```python
from build123d import *

# Parameters (mm, degrees)
SKETCH1_W           = 22.225
SKETCH1_H           = 17.4625
BOSS_EXTRUDE1_DEPTH = 50.8
CUT_EXTRUDE1_REACH  = 60.134
SKETCH2_R           = 2.032


with BuildPart() as part:
    # Sketch1 → Boss-Extrude1 (new body)
    with BuildSketch(Plane.XY):
        with Locations((11.1125, 8.73125)):
            Rectangle(SKETCH1_W, SKETCH1_H)
    extrude(amount=BOSS_EXTRUDE1_DEPTH)

    # Sketch2 → Cut-Extrude1 (cut, up to next)
    with BuildSketch(Plane.XZ, mode=Mode.PRIVATE) as cut_extrude1_sk1:
        with Locations(Location((11.1125, 44.45, 0), (0, 0, 270))):
            Circle(SKETCH2_R)
    cut_extrude1_tool1 = extrude(cut_extrude1_sk1.sketch, amount=-CUT_EXTRUDE1_REACH, mode=Mode.PRIVATE) & part.part
    # Sketch2 → Cut-Extrude1 (cut, up to next)
    with BuildSketch(Plane.XZ, mode=Mode.PRIVATE) as cut_extrude1_sk2:
        with Locations(Location((11.1125, 6.35, 0), (0, 0, 270))):
            Circle(SKETCH2_R)
    cut_extrude1_tool2 = extrude(cut_extrude1_sk2.sketch, amount=-CUT_EXTRUDE1_REACH, mode=Mode.PRIVATE) & part.part
    # Sketch2 → Cut-Extrude1 (cut, up to next)
    with BuildSketch(Plane.XZ, mode=Mode.PRIVATE) as cut_extrude1_sk3:
        Polygon((14.998644662, 25.4), (13.055572331, 28.7655), (9.169427669, 28.7655), (7.226355338, 25.4), (9.169427669, 22.0345), (13.055572331, 22.0345), align=None)
    cut_extrude1_tool3 = extrude(cut_extrude1_sk3.sketch, amount=-CUT_EXTRUDE1_REACH, mode=Mode.PRIVATE) & part.part
    add(cut_extrude1_tool1.solids().sort_by_distance((11.1125, 0, 44.45))[0], mode=Mode.SUBTRACT)
    add(cut_extrude1_tool2.solids().sort_by_distance((11.1125, 0, 6.35))[0], mode=Mode.SUBTRACT)
    add(cut_extrude1_tool3.solids().sort_by_distance((11.1125, 0, 25.4))[0], mode=Mode.SUBTRACT)


solid = part.part
```
Geometry check sheet. Reference: the model listing, model coordinates, mm. A direction names the side the tool comes from. Round coordinates to 2 decimals unless told otherwise and drop trailing zeros. Order: outer loops, then holes, each group sorted by start corner. A loop starts at its lowest first (then second) coordinate and runs counter-clockwise, first axis right, second up. Notation, with made-up numbers: (57.25, -20) - (74.25, -20) arc R26 cw to (74.25, -1) - close; hole circle Ø10 at (56, -4.5). An arc over 180 degrees is marked (long way). Use a Markdown table: item, result. Add a question column.
(1) Sectioned sample at B-B, the plane z = 6.35. Enter the section's corners in (x, y) (1 decimal), and give its area (3 significant figures).
(2) Material ranges on line 1 along Z through (x, y) = (11.25, 16); line 2 along X through (y, z) = (6.25, 6.35) (1 decimal); line 3 along Z through (x, y) = (9.5, 12.5), recorded low to high. Write a range as [from, to].
(3) Release check for a two-part mould opening along Z. For faces 1 (the flat face through (11, 9, 0)), 2 (the flat face through (0, 9, 25)), 3 (the flat face through (14.04, 8.61, 27.06)) record: pulls with the +Z half, pulls with the -Z half, needs draft (parallel to the pull), parting line crosses it, or undercut.
(4) Tool access check on faces 4 (the flat face through (22.225, 9, 25)), 5 (the flat face through (11, 9, 28.766)). Record the directions out of +Z, -Z, +X, -X, +Y, -Y that give a thin tool (end or side, any length) a straight path to the whole face; none if there is none.
(5) Sectioned sample at C-C, the plane y = 2.75. Count the separate pieces of the cut face and the enclosed holes in it, and give its area (3 significant figures).
(6) Sectioned sample at A-A, the plane x = 8. Enter the section's corners in (y, z).
Answers below:
| question | item | result |
|---|---|---|
| 1 | outline | (0, 0) - (9.1, 0) - (9.1, 17.5) - (0, 17.5) - close; (13.1, 0) - (22.2, 0) - (22.2, 17.5) - (13.1, 17.5) - close |
| 1 | area | 317 mm² |
| 2 | line 1 | [0, 4.32], [8.38, 22.03], [28.77, 42.42], [46.48, 50.8] |
| 2 | line 2 | [0, 9.1], [13.1, 22.2] |
| 2 | line 3 | [0, 5.11], [7.59, 22.03], [28.77, 43.21], [45.69, 50.8] |
| 3 | face 1 | pulls with the -Z half |
| 3 | face 2 | needs draft |
| 3 | face 3 | undercut |
| 4 | face 4 | +Z, -Z, +X, +Y, -Y |
| 4 | face 5 | +Y, -Y |
| 5 | separate pieces | 1 |
| 5 | enclosed holes | 3 |
| 5 | area | 1,060 mm² |
| 6 | outline | (0, 0) - (17.46, 0) - (17.46, 24.06) - (0, 24.06) - close; (0, 26.74) - (17.46, 26.74) - (17.46, 50.8) - (0, 50.8) - close |
